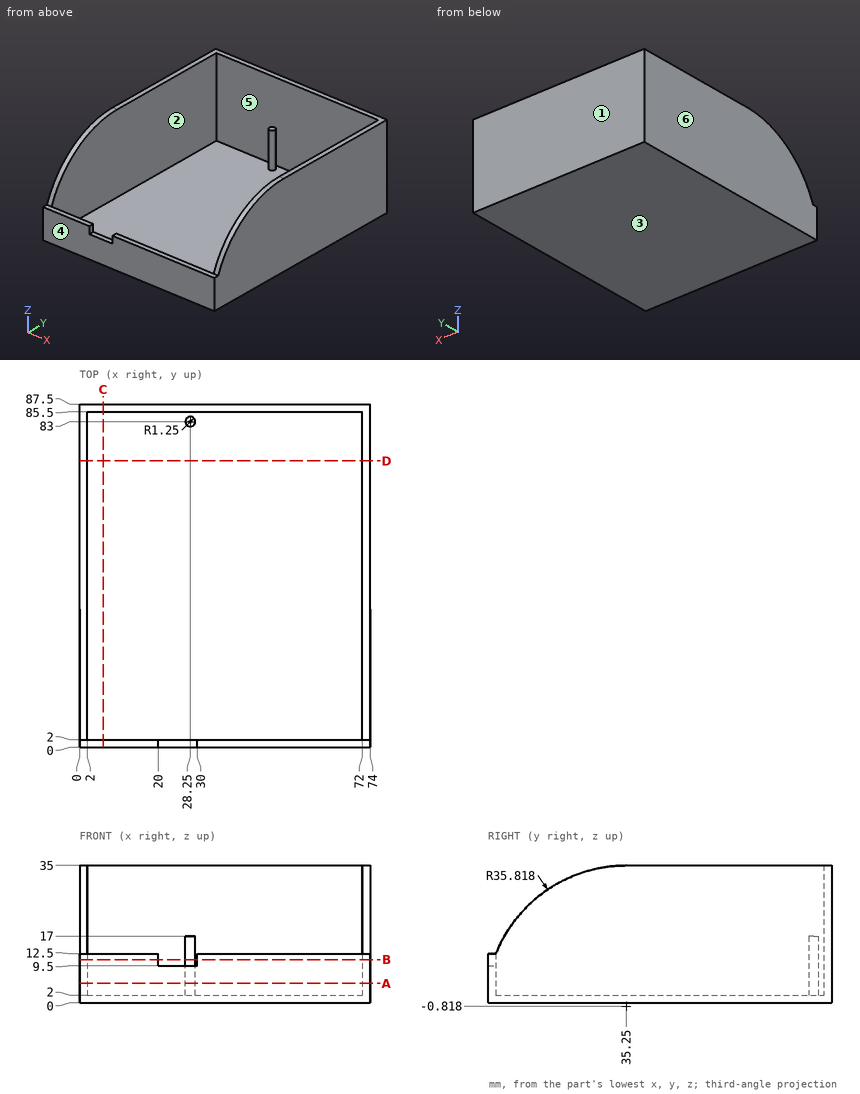
Design review of the part shown in the three views and the two pictorial views. Dimensions are in mm from the part's minimum x, y and z. A direction names the side the tool comes from. Round coordinates to 2 decimals unless told otherwise and drop trailing zeros. Write each loop counter-clockwise with the first axis right and the second up, starting at its lowest first coordinate (ties: lowest second). Pieces come first, ordered by that corner, then holes. Notation, with made-up numbers: (32.25, 71.5) -> (83.25, 71.5) arc R16 cw to (83.25, 76.5) -> close; hole circle Ø5 at (-32.75, -4.5). An arc over 180 degrees is marked (long way). Write item = value, one per line. Start each with the question number.
1) Clearance check with flat-ended pins moving along their axes: pin 1 (2 mm diameter, centred on x = 28, y = 83, fed in from +Z); pin 2 (4 mm diameter, centred on x = 31, z = 17.5, fed in from -Y); pin 3 (4 mm diameter, centred on x = 36.5, y = 57, fed in from +Z). State where each tip first meets the part, or that it passes through.
2) Take a section at B-B, the plane z = 11. State the section outline as (x, y) points.
3) Take a section at A-A, the plane z = 5. State the section outline as (x, y) points, plus the area to 3 significant figures.
4) Tool access review of the marked faces 5 and 6: name each direction out of +Z, -Z, +X, -X, +Y, -Y from which nothing blocks a thin tool from reaching the whole face with its end or side.
5) Wall thickness on probe 1 along X at (y, z) = (12.5, 19.5); probe 2 along Y at (x, z) = (49.5, 33); probe 3 along Z at (x, y) = (70, 22.5): over which ranges is each line inside the solid? List them lowest first. Write a range as from..to.
6) Take a section at D-D, the plane y = 73. State the section outline as (x, z) points, plus the area to 3 significant figures.
7) Mouldability with a two-part tool opening along Y and no side actions: class the marked faces 1, 2, 3 and 4 as +Y half, -Y half, draft (parallel to the pull), parting line (faces both ways), or undercut.
8) Take a section at C-C, the plane x = 6. State the section outline as (y, z) points, plus the area to 3 significant figures.
Results list:
q1.pin_1 = 17
q1.pin_2 = 82.05
q1.pin_3 = 2
q2.outline = (0, 0) -> (20, 0) -> (20, 2) -> (2, 2) -> (2, 85.5) -> (72, 85.5) -> (72, 2) -> (30, 2) -> (30, 0) -> (74, 0) -> (74, 87.5) -> (0, 87.5) -> close; (27, 83) arc R1.25 ccw to (29.5, 83) arc R1.25 ccw to (28.25, 84.25) arc R1.25 ccw to start
q3.outline = (0, 0) -> (74, 0) -> (74, 87.5) -> (0, 87.5) -> close; (27, 83) arc R1.25 ccw to (29.5, 83) arc R1.25 ccw to (28.25, 84.25) arc R1.25 ccw to start; hole (2, 2) -> (72, 2) -> (72, 85.5) -> (2, 85.5) -> close
q3.area = 635 mm²
q4.face_5 = +Z
q4.face_6 = +Z, -Z, -X, +Y, -Y
q5.probe_1 = 0..2, 72..74
q5.probe_2 = 85.5..87.5
q5.probe_3 = 0..2
q6.outline = (0, 0) -> (74, 0) -> (74, 35) -> (72, 35) -> (72, 2) -> (2, 2) -> (2, 35) -> (0, 35) -> close
q6.area = 280 mm²
q7.face_1 = +Y half
q7.face_2 = undercut
q7.face_3 = draft
q7.face_4 = -Y half
q8.outline = (0, 0) -> (87.5, 0) -> (87.5, 35) -> (85.5, 35) -> (85.5, 2) -> (2, 2) -> (2, 12.5) -> (0, 12.5) -> close
q8.area = 262 mm²
